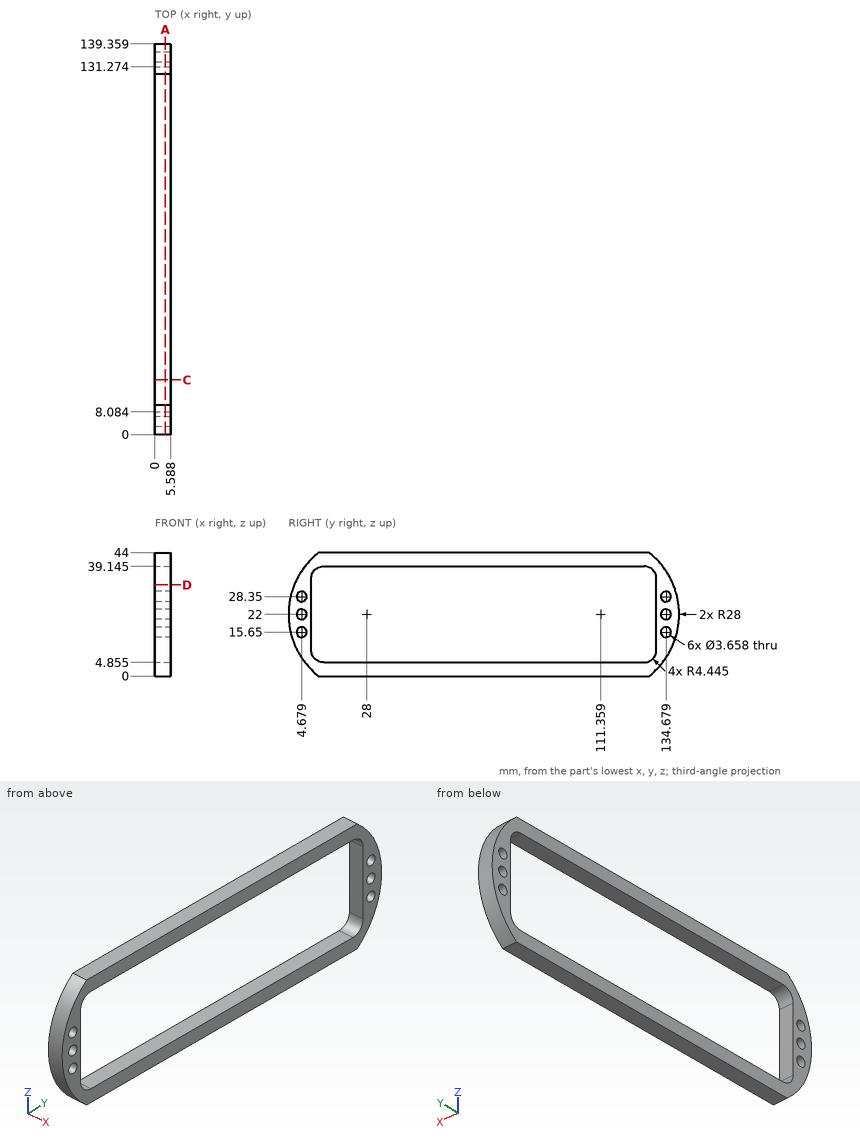
Design review of the part shown in the three views and the two pictorial views. Dimensions are in mm from the part's minimum x, y and z. Coordinates: 2 decimals unless noted, no trailing zeros. Loops run counter-clockwise (first coordinate to the right, second up) from the corner with the lowest first, then second, coordinate; pieces in that order, holes last. Notation, with made-up numbers: M -2.75,5.25 L 53.25,5.25 A19 ccw 53.25,19.25 Z; hole C 37.25,55.25 d10. An arc over 180 degrees is marked long. One line per question, with ' | ' between items.
(1) We need section C-C (y = 19.5). Give the boundary of the cut face in (x, z) (1 decimal).
Filled in:
outline: M 0,0 L 5.6,0 L 5.6,4.9 L 0,4.9 Z; M 0,39.1 L 5.6,39.1 L 5.6,44 L 0,44 Z
(2) For pin 1 Ø1 at (x, z) = (2.5, 17) entering from -Y; pin 2 Ø6 at (y, z) = (4.68, 28.35) entering from +X, all flat-tipped, find the tip position at first contact; note any pin that passes through.
Filled in:
pin 1: stops at y = 0.36 | pin 2: stops at x = 5.59
(3) Wall thickness on probe 1 along Z at (x, y) = (3.9, 102) (1 decimal); probe 2 along Y at (x, z) = (3.6, 15) (1 decimal); probe 3 along Y at (x, z) = (0.75, 24) (1 decimal): over which ranges is each line inside the solid? List them lowest first.
Filled in:
probe 1: z = 0 to 4.9, 39.1 to 44 | probe 2: y = 0.9 to 3, 6.4 to 8.1, 131.3 to 133, 136.4 to 138.5 | probe 3: y = 0.1 to 8.1, 131.3 to 139.3
(4) We need section D-D (z = 32.5). Give the boundary of the cut face in (x, y) (1 decimal).
Filled in:
outline: M 0,2 L 5.6,2 L 5.6,8.1 L 0,8.1 Z; M 0,131.3 L 5.6,131.3 L 5.6,137.3 L 0,137.3 Z
(5) We need section A-A (x = 3.75). Count the separate pieces of the cut face and the enclosed holes in it, and give its area (3 significant figures).
Filled in:
separate pieces: 1 | enclosed holes: 7 | area: 1,580 mm^2
